Here's how the part is built. I have some questions about the finished solid (model axes, mm). A direction names the side the tool comes from. Round coordinates to 2 decimals unless told otherwise and drop trailing zeros. Write each loop counter-clockwise with the first axis right and the second up, starting at its lowest first coordinate (ties: lowest second). Pieces come first, ordered by that corner, then holes. Notation, with made-up numbers: (-17.5, 29.5) -> (23.5, 29.5) arc R32 ccw to (23.5, 56.5) -> close; hole circle Ø2 at (67, 60). An arc over 180 degrees is marked (long way). Answer in a Markdown table with one row per item. Add a question column.
from build123d import *

# Parameters (mm, degrees)
SKETCH1_R           = 32
SKETCH1_R_2         = 18
BOSS_EXTRUDE1_DEPTH = 36
SKETCH2_R           = 21
SKETCH2_R_2         = 12
BOSS_EXTRUDE2_DEPTH = 24
SKETCH3_R           = 18
SKETCH3_R_2         = 12
BOSS_EXTRUDE3_DEPTH = 12
CUT_EXTRUDE1_DEPTH  = 131.234404057
BOSS_EXTRUDE4_DEPTH = 6


with BuildPart() as part:
    # Sketch1 → Boss-Extrude1 (new body)
    with BuildSketch(Plane(origin=(0, 0, 0), x_dir=(1, 0, 0), z_dir=(0, 1, 0))):
        with Locations(Location((0, 0, 0), (0, 0, 270))):
            Circle(SKETCH1_R)
        with Locations(Location((0, 0, 0), (0, 0, 270))):
            Circle(SKETCH1_R_2, mode=Mode.SUBTRACT)
    extrude(amount=BOSS_EXTRUDE1_DEPTH)



with BuildPart() as body_2:
    # Sketch2 → Boss-Extrude2 (new body)
    with BuildSketch(Plane(origin=(0, 0, 0), x_dir=(1, 0, 0), z_dir=(0, 1, 0))):
        with Locations(Location((-100, 0, 0), (0, 0, 270))):
            Circle(SKETCH2_R)
        with Locations(Location((-100, 0, 0), (0, 0, 270))):
            Circle(SKETCH2_R_2, mode=Mode.SUBTRACT)
    extrude(amount=BOSS_EXTRUDE2_DEPTH)


with BuildPart() as part_1:
    add(part.part)

    add(body_2.part)  # Boss-Extrude3 merges body 2
    # Sketch3 → Boss-Extrude3 (add)
    with BuildSketch(Plane.XZ):
        with BuildLine():
            Line((-102.31, 20.872563331), (-3.52, 31.80581079))
            ThreePointArc((-3.52, 31.80581079), (32, 0), (-3.52, -31.80581079))
            Line((-3.52, -31.80581079), (-102.31, -20.872563331))
            ThreePointArc((-102.31, -20.872563331), (-121, 0), (-102.31, 20.872563331))
        make_face()
        with Locations(Location((0, 0, 0), (0, 0, 90))):
            Circle(SKETCH3_R, mode=Mode.SUBTRACT)
        with Locations(Location((-100, 0, 0), (0, 0, 270))):
            Circle(SKETCH3_R_2, mode=Mode.SUBTRACT)
    extrude(amount=-BOSS_EXTRUDE3_DEPTH)

    # Sketch4 → Cut-Extrude1 (cut, through all)
    with BuildSketch(Plane(origin=(0, 36, 0), x_dir=(1, 0, 0), z_dir=(0, 1, 0))):
        with BuildLine():
            Line((-23.000562748, 6), (-16.970562748, 6))
            ThreePointArc((-16.970562748, 6), (-18, 0), (-16.970562748, -6))
            Line((-16.970562748, -6), (-23.000562748, -6))
            Line((-23.000562748, -6), (-23.000562748, 6))
        make_face()
    extrude(amount=-CUT_EXTRUDE1_DEPTH, mode=Mode.SUBTRACT)

    # Sketch5 → Boss-Extrude4 (add, symmetric)
    with BuildSketch(Plane.XY):
        Polygon((-80.173004722, 12), (-80.173004722, 24), (-79, 24), (-32, 36), (-30.333655542, 36), (-30.333655542, 12), align=None)
    extrude(amount=BOSS_EXTRUDE4_DEPTH, both=True)


solid = part_1.part
Item 1: On a 3-axis mill with a long thin cutter (end or side, diameter ignored), from which of +Z, -Z, +X, -X, +Y, -Y can I reach the whole of each face in a straight line? I mean faces 4 (the cylindrical face through (31.973, 21.748, 1.323)), 5 (the flat face through (-55, 22, 6)), 6 (the flat face through (-52, 12, -16)), 7 (the flat face through (-23.001, 18, 0)). Say none if no direction works.
Item 2: For P1, Ø13, axis at y = 12, z = -0.5, coming from the +X side; P2, Ø3, axis at x = -19.5, y = 12, coming from the -Z side; P3, Ø1.5, axis at x = -19.5, y = 5.5, coming from the +Z side, each with a flat end and sliding along its axis, tell me the tip position at first contact or that it passes through.
Item 3: If we section it at D-D on y = 32.5: Please give me the cut outline in (x, z), then the cut area to 3 significant figures.
Item 4: If we mould it in two halves opening along X, with no side actions, what happens to faces 1 (the flat face through (-52.223, 5.916, -26.416)), 2 (the cylindrical face through (-96.396, 11.832, 11.446)), 3 (the flat face through (14, 36, -14))? For each: pulls with the +X half, pulls with the -X half, needs draft (parallel to the pull), parting line crosses it, or undercut.
Item 5: If we section it at A-A on x = 0: Please give me the cut outline in (y, z).
Item 6: I need wall thicknesses on line 1 along X through (y, z) = (2, -0.5); line 2 along Z through (x, y) = (0, 11); line 3 along X through (y, z) = (21.5, -14). Which ranges of each line are inside material? Lowest first, please. Write a range as from..to.
Item 7: If we section it at C-C on y = 15.5: Please give me the cut outline in (x, z).
Item 8: If we section it at B-B on z = 0: Please give me the cut outline in (x, y).
Results list:
| question | item | result |
|---|---|---|
| 1 | face 4 | +Y |
| 1 | face 5 | +Z, +Y |
| 1 | face 6 | -Z, +Y |
| 1 | face 7 | +Y, -Y |
| 2 | P1 | x = 32 |
| 2 | P2 | z = -30.2 |
| 2 | P3 | z = 30.12 |
| 3 | outline | (-45.71, -6) -> (-31.43, -6) arc R32 ccw (long way) to (-31.43, 6) -> (-45.71, 6) -> close; hole (-23, -6) -> (-16.97, -6) arc R18 ccw (long way) to (-16.97, 6) -> (-23, 6) -> close |
| 3 | area | 2,300 mm² |
| 4 | face 1 | pulls with the -X half |
| 4 | face 2 | undercut |
| 4 | face 3 | needs draft |
| 5 | outline | (0, -32) -> (36, -32) -> (36, -18) -> (0, -18) -> close; (0, 18) -> (36, 18) -> (36, 32) -> (0, 32) -> close |
| 6 | line 1 | -120.99..-111.99, -88.01..-23, 17.99..32 |
| 6 | line 2 | -32..-18, 18..32 |
| 6 | line 3 | -115.65..-84.35, -28.77..-11.31, 11.31..28.77 |
| 7 | outline | (-79.88, -6) -> (-31.43, -6) arc R32 ccw (long way) to (-31.43, 6) -> (-79.88, 6) arc R21 ccw (long way) to start; hole circle Ø24 at (-100, 0); hole (-23, -6) -> (-16.97, -6) arc R18 ccw (long way) to (-16.97, 6) -> (-23, 6) -> close |
| 8 | outline | (-121, 0) -> (-112, 0) -> (-112, 24) -> (-121, 24) -> close; (-88, 0) -> (-23, 0) -> (-23, 36) -> (-32, 36) -> (-79, 24) -> (-88, 24) -> close; (18, 0) -> (32, 0) -> (32, 36) -> (18, 36) -> close |
